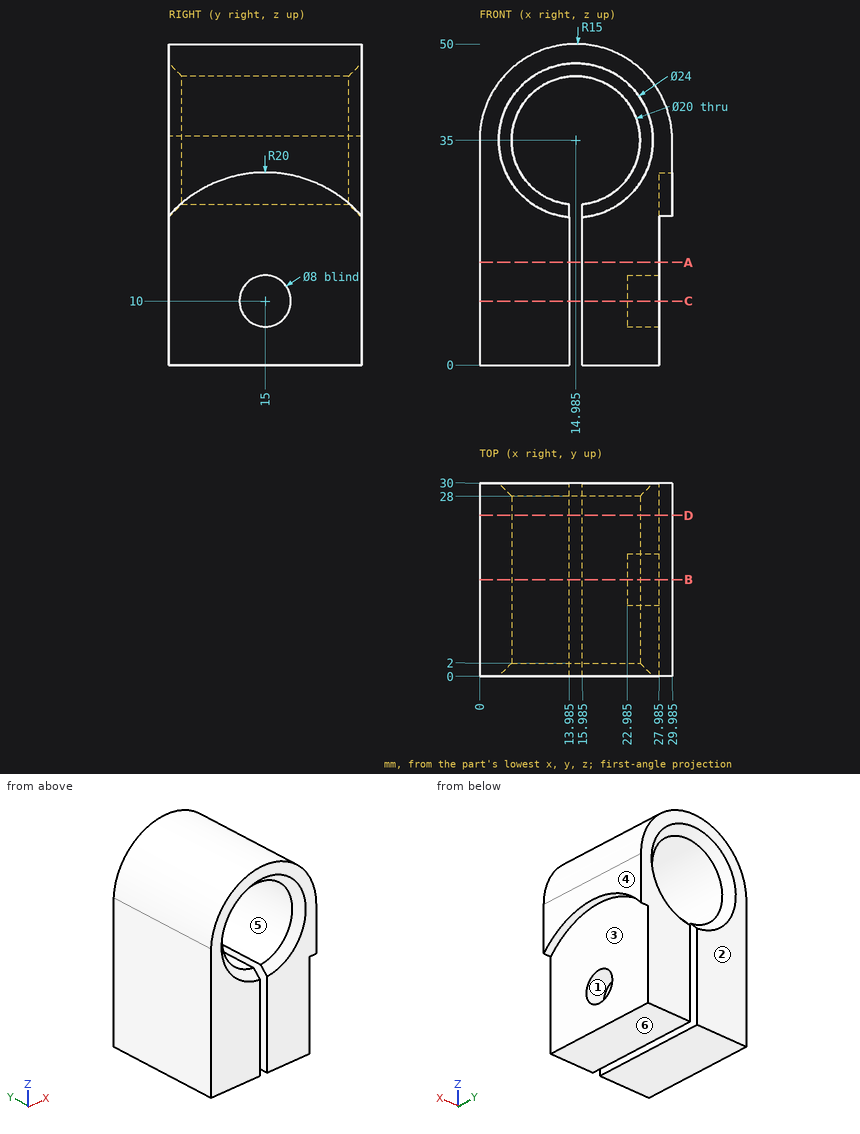
Answer from the drawing. Dimensions are ordinates in mm from the lowest x, y and z of the part. A direction names the side the tool comes from. Round coordinates to 2 decimals unless told otherwise and drop trailing zeros. Loops run counter-clockwise (first coordinate to the right, second up) from the corner with the lowest first, then second, coordinate; pieces in that order, holes last.
1) A cutting plane is placed at D-D on y = 25. Determine the outline of the cut face in (x, z) (1 decimal).
Outcome:
outline: (0, 0) - (14, 0) - (14, 25.1) arc R10 cw (long way) to (16, 25.1) - (16, 0) - (28, 0) - (28, 27.3) - (30, 27.3) - (30, 35) arc R15 ccw to (0, 35.7) - close
2) Given P1, Ø9, axis at y = 10.5, z = 17, coming from the +X side (3 decimals); P2, Ø10, axis at x = 19, z = 34, coming from the +Y side; P3, Ø3, axis at x = 15.5, z = 44, coming from the +Y side; P4, Ø3, axis at x = 9.5, y = 17.5, coming from the +Z side, each flat-ended and moving along its own axis, determine where each tip first touches the part or whether it passes through.
Outcome:
P1: stops at x = 27.985
P2: passes through
P3: stops at y = 28.51
P4: stops at z = 49.46
3) A cutting plane is placed at A-A on z = 16. Determine the outline of the cut face in (x, y) (3 decimals), plus the area to 3 significant figures.
Outcome:
outline: (0, 0) - (13.985, 0) - (13.985, 30) - (0, 30) - close; (15.985, 0) - (27.985, 0) - (27.985, 30) - (15.985, 30) - close
area: 780 mm2
4) A cutting plane is placed at B-B on y = 15. Determine the outline of the cut face in (x, z) (3 decimals).
Outcome:
outline: (0, 0) - (13.985, 0) - (13.985, 25.05) arc R10 cw (long way) to (15.985, 25.05) - (15.985, 0) - (27.985, 0) - (27.985, 6) - (22.985, 6) - (22.985, 14) - (27.985, 14) - (27.985, 30) - (29.985, 30) - (29.985, 35) arc R15 ccw to (0, 35.67) - close
5) For the marked faces 1, 2 and 3, determine the directions among +Z, -Z, +X, -X, +Y, -Y from which every point of the face is accessible in a straight line to the end or side of a thin tool.
Outcome:
face 1: +X
face 2: +Z, -Z, +X, -X, +Y
face 3: -Z, +X
6) A cutting plane is placed at C-C on z = 10. Determine the outline of the cut face in (x, y) (3 decimals), plus the area to 3 significant figures.
Outcome:
outline: (0, 0) - (13.985, 0) - (13.985, 30) - (0, 30) - close; (15.985, 0) - (27.985, 0) - (27.985, 11) - (22.985, 11) - (22.985, 19) - (27.985, 19) - (27.985, 30) - (15.985, 30) - close
area: 740 mm2
7) Consider line 1 (X direction, y = 6.25, z = 11) (3 decimals); line 2 (X direction, y = 20.75, z = 35) (3 decimals); line 3 (Z direction, x = 24.2, y = 15). Determine where each line is inside the solid, lowest interval first.
Outcome:
line 1: x = 0 to 13.985, 15.985 to 27.985
line 2: x = 0 to 4.985, 24.985 to 29.985
line 3: z = 0 to 6, 14 to 31.12, 38.88 to 46.84
8) For a pull along Z with two mould halves and no side action, classify the marked faces 4, 5 and 6 as released by +Z, released by -Z, zero draft, split by the parting line, or undercut.
Outcome:
face 4: zero draft
face 5: undercut
face 6: released by -Z
